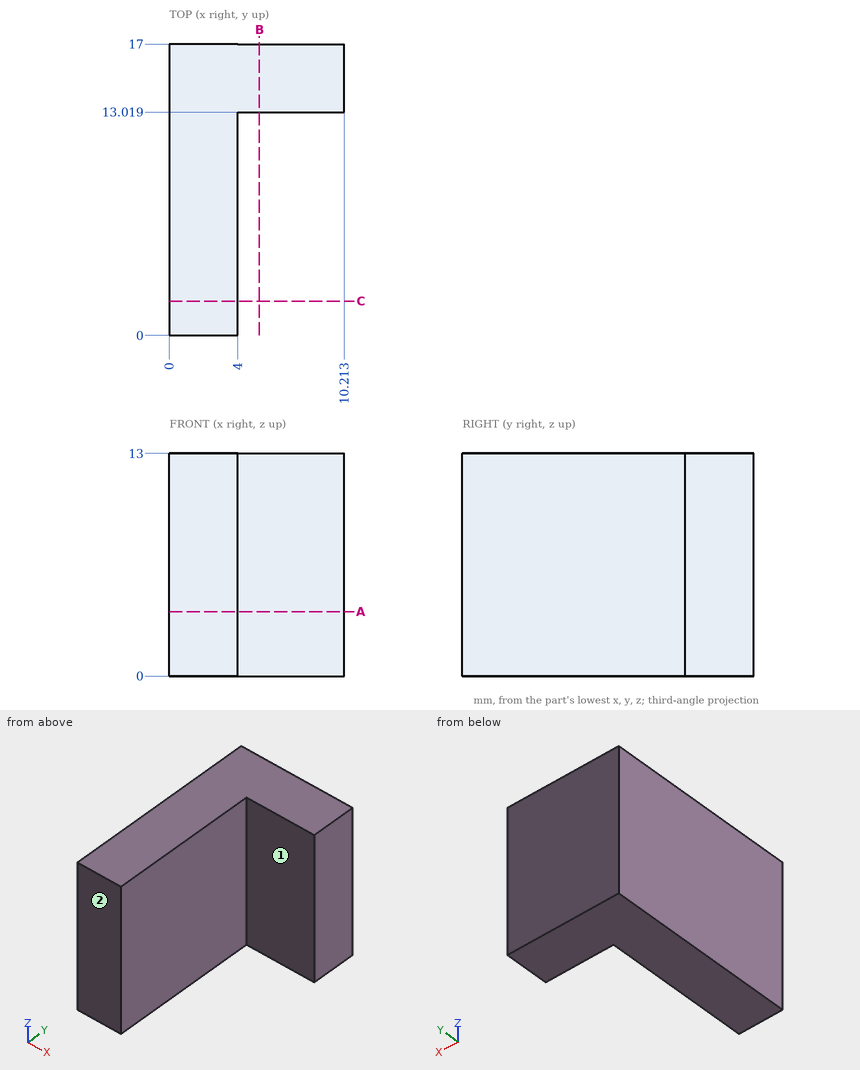
Geometry: see drawing. Coordinates: mm, zero at the bounding-box minimum. A direction names the side the tool comes from. Give positions to 0.01 mm unless a question says otherwise; leave off trailing zeros. Loops run counter-clockwise (first coordinate to the right, second up) from the corner with the lowest first, then second, coordinate; pieces in that order, holes last. Notation, with made-up numbers: (1, 31) -> (32, 31) arc R28 cw to (32, 61) -> close; hole circle Ø8 at (-34.5, 35.25). An arc over 180 degrees is marked (long way). Use CSV: the item, a comma, the result in double quotes.
(1) Cut plane A-A (z = 3.75). Output: boundary loops of the cut face in (x, y).
From the geometry:
outline,"(0, 0) -> (4, 0) -> (4, 13.02) -> (10.21, 13.02) -> (10.21, 17) -> (0, 17) -> close"
(2) Cut plane B-B (x = 5.25). Output: boundary loops of the cut face in (y, z).
From the geometry:
outline,"(13.02, 0) -> (17, 0) -> (17, 13) -> (13.02, 13) -> close"
(3) Ray query, line 1 along Y through (x, z) = (6.5, 3.5); line 2 along X through (y, z) = (2.25, 9.5). Return the intervals inside material, ascending. Write a range as [from, to].
From the geometry:
line 1,"[13.02, 17]"
line 2,"[0, 4]"
(4) Cut plane C-C (y = 2). Output: boundary loops of the cut face in (x, z), plus the area to 3 significant figures.
From the geometry:
outline,"(0, 0) -> (4, 0) -> (4, 13) -> (0, 13) -> close"
area,"52.0 mm^2"
(5) Access query for the marked faces 1 and 2. Directions: +Z, -Z, +X, -X, +Y, -Y. A direction counts if a zero-diameter tool reaches every point of the face in a straight line with its end or side. Return the directions, or none.
From the geometry:
face 1,"+Z, -Z, +X, -Y"
face 2,"+Z, -Z, +X, -X, -Y"
(6) First-contact query: P1, Ø4, axis at x = 5.5, y = 8.5, coming from the +Z side; P2, Ø5, axis at x = 7.5, z = 6.5, coming from the -Y side. Flat tips, straight axial feed; report the tip coordinate or a pass-through.
From the geometry:
P1,"z = 13"
P2,"y = 13.02"
